```python
from build123d import *

# Parameters (mm, degrees)
F1_DEPTH = 3


with BuildPart() as f1:
    # F0 (on Top) → F1 (new body)
    with BuildSketch(Plane.XY):
        with BuildLine():
            ThreePointArc((-34.25, 2.5), (-36.75, 0), (-34.25, -2.5))
            Line((-34.25, -2.5), (-29.25, -2.5))
            ThreePointArc((-29.25, -2.5), (-26.75, 0), (-29.25, 2.5))
            Line((-29.25, 2.5), (-34.25, 2.5))
        make_face()
        with BuildLine():
            Line((0, -7.5), (0, 7.5))
            Line((0, 7.5), (-34.5, 7.5))
            ThreePointArc((-34.5, 7.5), (-39.803301, 5.303301), (-42, 0))
            ThreePointArc((-42, 0), (-39.803301, -5.303301), (-34.5, -7.5))
            Line((-34.5, -7.5), (0, -7.5))
        make_face()
        with BuildLine():
            Line((-29.25, -2.5), (-34.25, -2.5))
            ThreePointArc((-34.25, -2.5), (-36.75, 0), (-34.25, 2.5))
            Line((-34.25, 2.5), (-29.25, 2.5))
            ThreePointArc((-29.25, 2.5), (-26.75, 0), (-29.25, -2.5))
        make_face(mode=Mode.SUBTRACT)
        with BuildLine():
            Line((34.5, 7.5), (0, 7.5))
            Line((0, 7.5), (0, -7.5))
            Line((0, -7.5), (34.5, -7.5))
            ThreePointArc((34.5, -7.5), (39.803301, -5.303301), (42, 0))
            ThreePointArc((42, 0), (39.803301, 5.303301), (34.5, 7.5))
        make_face()
        with BuildLine():
            ThreePointArc((29.25, -2.5), (26.75, 0), (29.25, 2.5))
            Line((29.25, 2.5), (34.25, 2.5))
            ThreePointArc((34.25, 2.5), (36.75, 0), (34.25, -2.5))
            Line((34.25, -2.5), (29.25, -2.5))
        make_face(mode=Mode.SUBTRACT)
    extrude(amount=F1_DEPTH)


solid = f1.part
```
CAD build for the part. Positions are in the model's coordinates, mm. A direction names the side the tool comes from. Give positions to 0.01 mm unless a question says otherwise; leave off trailing zeros. Loops run counter-clockwise (first coordinate to the right, second up) from the corner with the lowest first, then second, coordinate; pieces in that order, holes last. Notation, with made-up numbers: M 6,-33.75 L 36,-33.75 A11 cw 36,-26.75 Z; hole C 4,-5 d7. An arc over 180 degrees is marked long. Use one line per item in the form item = value.
Item 1: Which spindle directions (+Z, -Z, +X, -X, +Y, -Y) get a long thin tool onto all of the face, cutting with end or side? Do faces 4 (the face through (0, -7.5, 1)), 5 (the face through (26.75, -0.05, 1.48)). Say none if no direction does.
Determined:
face_4 = +Z, -Z, +X, -X, -Y
face_5 = +Z, -Z
Item 2: Slice it at B-B (y = -4.75). List the corners of the cut face in (x, z).
Determined:
outline = M -40.3,0 L 40.3,0 L 40.3,3 L -40.3,3 Z
Item 3: Slice it at C-C (y = 3.5). List the corners of the cut face in (x, z), plus the area to 3 significant figures.
Determined:
outline = M -41.13,0 L 41.13,0 L 41.13,3 L -41.13,3 Z
area = 247 mm2
Item 4: Drill centre lines: probe 1 along X at (y, z) = (0.25, 2.25); probe 2 along Y at (x, z) = (-31.5, 2.65); probe 3 along X at (y, z) = (-1.25, 0.5). Where is each one in solid material? Low to high. Write a range as from..to.
Determined:
probe_1 = -42..-36.74, -26.76..26.76, 36.74..42
probe_2 = -7.5..-2.5, 2.5..7.5
probe_3 = -41.9..-36.42, -27.08..27.08, 36.42..41.9
Item 5: Slice it at A-A (z = 1.3). List the corners of the cut face in (x, y).
Determined:
outline = M -34.5,-7.5 L 34.5,-7.5 A7.5 ccw 34.5,7.5 L -34.5,7.5 A7.5 ccw Z; hole M -34.25,-2.5 L -29.25,-2.5 A2.5 ccw -29.25,2.5 L -34.25,2.5 A2.5 ccw Z; hole M 29.25,-2.5 L 34.25,-2.5 A2.5 ccw 34.25,2.5 L 29.25,2.5 A2.5 ccw Z
Item 6: Two-plate mould, pull along Y, no slides. Class faces 1 (the face through (-32, 2.5, 1)), 2 (the face through (0, 7.5, 1)), 3 (the face through (-1, 0, 0)): pulls with the +Y half, pulls with the -Y half, needs draft (parallel to the pull), parting line crosses it, or undercut.
Determined:
face_1 = undercut
face_2 = pulls with the +Y half
face_3 = needs draft
Item 7: Flat gauge pins, fed straight in: pin 1 (6 mm diameter, centred on x = 0.5, y = 2, fed in from -Z); pin 2 (1 mm diameter, centred on y = -1, z = 2, fed in from +X). Where does each tip first touch, or does it go through?
Determined:
pin_1 = 0
pin_2 = 41.98
